Autodesk Inventor part; units mm, degrees
ref_plane "YZ Plane" through (0, 0, 0) normal (1, 0, 0) x (0, 1, 0)
ref_plane "XZ Plane" through (0, 0, 0) normal (0, 1, 0) x (-1, 0, 0)
ref_plane "XY Plane" through (0, 0, 0) normal (0, 0, 1) x (1, 0, 0)
sketch "Sketch1" plane through (0, 0, 0) normal (0, 0, 1) x (1, 0, 0)
  circle A0 centre (47.5, -34.875) radius 2.5
  circle A1 centre (47.5, 50.125) radius 2.5
  circle A2 centre (47.5, 35.125) radius 2.5
  circle A3 centre (47.5, -49.875) radius 2.5
  line L0 (50, -60) -> (52.5, -62.5)
  line L1 (52.5, -62.5) -> (52.5, -15)
  line L2 (52.5, -15) -> (37.5, -15)
  line L3 (37.5, -15) -> (37.5, -40)
  line L4 (37.5, -40) -> (27.5, -50)
  line L5 (27.5, -50) -> (-27.5, -50)
  line L6 (-27.5, -50) -> (-27.5, 50)
  line L7 (-27.5, 50) -> (27.5, 50)
  line L8 (27.5, 50) -> (37.5, 40)
  line L9 (37.5, 40) -> (37.5, 15)
  line L10 (37.5, 15) -> (52.5, 15)
  line L11 (52.5, 15) -> (52.5, 62.5)
  line L12 (52.5, 62.5) -> (50, 60)
  line L13 (50, 60) -> (-47.5, 60)
  line L14 (-57.5, 50) -> (-57.5, -50)
  line L15 (-47.5, -60) -> (50, -60)
  line L16 (-47.5, 60) -> (37.5, 60)
  line L17 (37.5, -60) -> (-47.5, -60)
  line L18 (-57.5, -50) -> (-57.5, 50)
  line L19 (0, 0) -> (31.4372, 0) construction
  line L20 (42.5, -54.9524) -> (47.5, -54.9524)
  line L21 (52.5, -49.9524) -> (52.5, -49.9524)
  line L22 (47.5, -44.9524) -> (42.5, -44.9524)
  arc A4 (52.5, -49.9524) -> (47.5, -44.9524) centre (47.5, -49.9524) ccw
  arc A5 (47.5, -54.9524) -> (52.5, -49.9524) centre (47.5, -49.9524) ccw
  line L23 (42.5, -54.9524) -> (42.5, -55)
  line L24 (42.5, 30) -> (47.5, 30)
  line L25 (47.5, 40) -> (42.5, 40)
  arc A6 (52.5, 35) -> (47.5, 40) centre (47.5, 35) ccw
  arc A7 (47.5, 30) -> (52.5, 35) centre (47.5, 35) ccw
  line L26 (42.5, 55) -> (42.5, 40)
  line L27 (42.5, 30) -> (42.5, -44.9524)
  line L28 (-27.5, 40) -> (37.5, 40)
  line L29 (37.5, 40) -> (37.5, -40)
  line L30 (37.5, -40) -> (-27.5, -40)
  line L31 (-27.5, -40) -> (-27.5, 40)
  line L32 (-57.5, 50) -> (-47.5, 60)
  line L33 (-57.5, -50) -> (-47.5, -60)
  line L34 (37.5, 60) -> (42.5, 55)
  line L35 (37.5, -60) -> (42.5, -55)
  circle A8 centre (-47.5, -50) radius 2.5
  circle A9 centre (35, 52.5) radius 2.5
  circle A10 centre (35, -52.5) radius 2.5
  circle A11 centre (-47.5, 50) radius 2.5
  line L36 (-57.5, -50) -> (-47.5, -60)
  line L37 (-47.5, 60) -> (-57.5, 50)
  point P0 (-57.5, 60)
  point P1 (42.5, -60)
  point P2 (42.5, 60)
  point P3 (-57.5, -60)
  point P4 (52.5, -44.9524)
  point P5 (52.5, -54.9524)
  point P6 (-57.5, 50)
  point P7 (-57.5, -50)
  point P8 (-27.5, -40)
  dimension "d2" = 10
  dimension "d3" = 10
  dimension "d4" = 10
  dimension "d5" = 5
  dimension "d6" = 5
  dimension "d7" = 5
  dimension "d8" = 5
  dimension "d9" = 30
  dimension "d10" = 10
  dimension "d11" = 10
  dimension "d12" = 10
  dimension "d13" = 10
  dimension "d14" = 10
  dimension "d15" = 5
  dimension "d16" = 5
  dimension "d17" = 5
  dimension "d18" = 5
extrude "Extrusion1" add sketch "Sketch1" along normal blind 5 contours L15 L33 L14 L32 L13 L34 L26 L25 A6 A7 L24 L27 L10 L9 L8 L7 L6 L5 L4 L3 L2 L22 A4 A5 L20 L23 L35 | L2 L29 L10 L27 | L4 L5 L6 L30 | L28 L6 L7 L8 | A8 | A9 | A10 | A11
sketch "Sketch2" plane through (0, 0, 5) normal (0, 0, 1) x (1, 0, 0)
  line L0 (37.5, 60) -> (-47.5, 60)
  line L1 (42.5, 40) -> (42.5, 55)
  line L2 (37.5, 40) -> (37.5, -40)
  line L3 (37.5, 0) -> (-27.5, 0) construction
  line L4 (-27.5, -40) -> (-27.5, 40)
  line L5 (-57.5, 50) -> (-57.5, -50)
  point P0 (0, 0)
  point P1 (-47.5, 50)
  point P2 (35, 52.5)
  point P3 (35, -52.5)
  point P4 (-27.5, -50)
  point P5 (-27.5, 50)
  point P6 (-47.5, -50)
  dimension "d21" = 7.5
  dimension "d22" = 7.5
  dimension "d23" = 10
  dimension "d24" = 10
hole "Hole1" at (-47.5, 50, 5) at (35, 52.5, 5) at (35, -52.5, 5) at (-47.5, -50, 5) direction (0, 0, -1) diameter 5 end through all
properties part number "Tapa" material "MDF Medium Density Fiberboard"
Model file for the job. Use its own axes, mm. A direction names the side the tool comes from. Give positions to 0.01 mm unless a question says otherwise; leave off trailing zeros. Loops run counter-clockwise (first coordinate to the right, second up) from the corner with the lowest first, then second, coordinate; pieces in that order, holes last.
1) Pull direction Y, two halves, no side cores. Call faces 1 (the flat face through (-52.6, -54.9, 2.5)), 2 (the cylindrical face through (52.5, 35.1, 2.5)), 3 (the flat face through (-52.6, 54.9, 2.5)), 4 (the flat face through (-57.5, 1, 2)): +Y half, -Y half, draft (parallel to the pull), parting line (faces both ways), or undercut.
2) Saw through at B-B (y = -5). Write the cut outline in (x, z).
3) Saw through at A-A (x = 35). Write the cut outline in (y, z).
4) Wall check: line 1 (Y direction, x = 35, z = 3.75); line 2 (Y direction, x = -47.5, z = 2.9); line 3 (Y direction, x = 47.5, z = 2.8) (3 decimals). Give the ranges that are in metal, low to high.
5) Flat gauge pins, fed straight in: pin 1 Ø4.5 at (x, y) = (47.5, -49.875) entering from -Z; pin 2 Ø2.5 at (x, z) = (44.5, 1.5) entering from +Y; pin 3 Ø1.5 at (y, z) = (11.5, 3) entering from +X; pin 4 Ø2.5 at (x, z) = (45.5, 2.5) entering from -Y. Where does each tip first touch, or does it go through?
6) Tool access for faces 5 (the flat face through (45, -54.952, 2)), 6 (the flat face through (45, 30, 2)), 7 (the flat face through (5, -40, 2)): list every direction of +Z, -Z, +X, -X, +Y, -Y with a clear straight run to the whole face (end or side of a thin tool).
7) Saw through at D-D (y = 41.5). Write the cut outline in (x, z).
8) Saw through at C-C (z = 1.6). Write the cut outline in (x, y) (3 decimals), plus the area to 3 significant figures.
Answer block:
1. face 1: -Y half
1. face 2: undercut
1. face 3: +Y half
1. face 4: draft
2. outline: (-57.5, 0) - (-27.5, 0) - (-27.5, 5) - (-57.5, 5) - close; (37.5, 0) - (42.5, 0) - (42.5, 5) - (37.5, 5) - close
3. outline: (-60, 0) - (-55, 0) - (-55, 5) - (-60, 5) - close; (-50, 0) - (-40, 0) - (-40, 5) - (-50, 5) - close; (40, 0) - (50, 0) - (50, 5) - (40, 5) - close; (55, 0) - (60, 0) - (60, 5) - (55, 5) - close
4. line 1: y = -60 to -55, -50 to -40, 40 to 50, 55 to 60
4. line 2: y = -60 to -52.5, -47.5 to 47.5, 52.5 to 60
4. line 3: y = -54.952 to -52.375, -47.375 to -44.952, 30 to 32.625, 37.625 to 40
5. pin 1: passes through
5. pin 2: stops at y = 40
5. pin 3: stops at x = 42.5
5. pin 4: stops at y = -54.95
6. face 5: +Z, -Z, +X, -Y
6. face 6: +Z, -Z, +X
6. face 7: +Z, -Z
7. outline: (-57.5, 0) - (42.5, 0) - (42.5, 5) - (-57.5, 5) - close
8. outline: (-57.5, -50) - (-47.5, -60) - (37.5, -60) - (42.5, -55) - (42.5, -54.952) - (47.5, -54.952) arc R5 ccw to (47.5, -44.952) - (42.5, -44.952) - (42.5, 30) - (47.5, 30) arc R5 ccw to (47.5, 40) - (42.5, 40) - (42.5, 55) - (37.5, 60) - (-47.5, 60) - (-57.5, 50) - close; hole circle Ø5 at (-47.5, -50); hole circle Ø5 at (-47.5, 50); hole (-27.5, -40) - (37.5, -40) - (37.5, 40) - (-27.5, 40) - close; hole circle Ø5 at (35, -52.5); hole circle Ø5 at (35, 52.5); hole circle Ø5 at (47.5, -49.875); hole circle Ø5 at (47.5, 35.125)
8. area: 6,740 mm2
